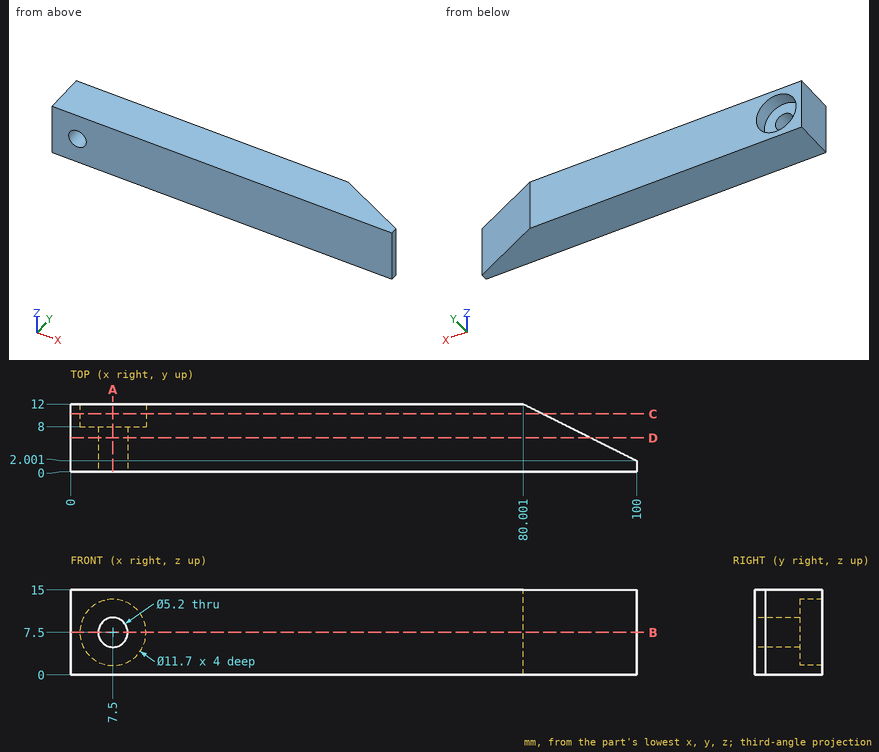
Can you work these out from the drawing? Everything is in mm from the part's minimum corner. Give positions to 0.01 mm unless a question says otherwise; leave off trailing zeros. Loops run counter-clockwise (first coordinate to the right, second up) from the corner with the lowest first, then second, coordinate; pieces in that order, holes last. Notation, with made-up numbers: M -39.5,12.5 L -32.5,12.5 A15 ccw -32.5,29.5 Z; hole C 34,-10.5 d8. An arc over 180 degrees is marked long. Use CSV: the item, a comma, the result in double quotes. Start each with the question number.
1. For P1, Ø1, axis at y = 7, z = 5, coming from the +X side, with a flat end and sliding along its axis, tell me the tip position at first contact or that it passes through.
2. Imagine slicing it at B-B, the plane z = 7.5. Write out the boundary of the cut face in (x, y).
3. Imagine slicing it at D-D, the plane y = 6. Write out the boundary of the cut face in (x, z).
4. If I drill on L1, parallel to Z at x = 7.5, y = 10.35; L2, parallel to X at y = 3.5, z = 7.5 (1 decimal); L3, parallel to X at y = 11, z = 11 (1 decimal), over which ranges is the centre line in solid material (lowest first)?
5. Imagine slicing it at A-A, the plane x = 7.5. Write out the boundary of the cut face in (y, z).
6. Imagine slicing it at C-C, the plane y = 10.25. Write out the boundary of the cut face in (x, z), plus the area to 4 significant figures.
Response values:
1,P1,"x = 91"
2,outline,"M 0,0 L 4.9,0 L 4.9,8 L 1.65,8 L 1.65,12 L 0,12 Z; M 10.1,0 L 100,0 L 100,2 L 80,12 L 13.35,12 L 13.35,8 L 10.1,8 Z"
3,outline,"M 0,0 L 92,0 L 92,15 L 0,15 Z; hole C 7.5,7.5 d5.2"
4,L1,"0 to 1.65, 13.35 to 15"
4,L2,"0 to 4.9, 10.1 to 97"
4,L3,"0 to 2.8, 12.2 to 82"
5,outline,"M 0,0 L 12,0 L 12,1.65 L 8,1.65 L 8,4.9 L 0,4.9 Z; M 0,10.1 L 8,10.1 L 8,13.35 L 12,13.35 L 12,15 L 0,15 Z"
6,outline,"M 0,0 L 83.5,0 L 83.5,15 L 0,15 Z; hole C 7.5,7.5 d11.7"
6,area,"1,145 mm^2"
